```python
from build123d import *

# Parameters (mm, degrees)
F1_DEPTH = 7.25
F2_R     = 0.5


with BuildPart() as f1:
    # F0 (on Top) → F1 (new body, symmetric)
    with BuildSketch(Plane.XY):
        with BuildLine():
            ThreePointArc((-6.9704381548, 3.1520615364), (-5, 0), (-6.9704381548, -3.1520615364))
            ThreePointArc((-6.9704381548, -3.1520615364), (-5.4093668761, -5.4093668761), (-3.1520615364, -6.9704381548))
            ThreePointArc((-3.1520615364, -6.9704381548), (0, -5), (3.1520615364, -6.9704381548))
            ThreePointArc((3.1520615364, -6.9704381548), (5.4093668761, -5.4093668761), (6.9704381548, -3.1520615364))
            ThreePointArc((6.9704381548, -3.1520615364), (5, 0), (6.9704381548, 3.1520615364))
            ThreePointArc((6.9704381548, 3.1520615364), (5.4093668761, 5.4093668761), (3.1520615364, 6.9704381548))
            ThreePointArc((3.1520615364, 6.9704381548), (0, 5), (-3.1520615364, 6.9704381548))
            ThreePointArc((-3.1520615364, 6.9704381548), (-5.4093668761, 5.4093668761), (-6.9704381548, 3.1520615364))
        make_face()
    extrude(amount=F1_DEPTH, both=True)

    # F2
    f2_edges = [f1.edges().sort_by_distance(p)[0] for p in [
        (-3.152062, 6.970438, 0),
        (-6.970438, 3.152062, 0),
        (-6.970438, -3.152062, 0),
        (-3.152062, -6.970438, 0),
        (3.152062, -6.970438, 0),
        (6.970438, -3.152062, 0),
        (6.970438, 3.152062, 0),
        (3.152062, 6.970438, 0),
    ]]
    fillet(f2_edges, radius=F2_R)

    # F3 (on Right) → F4 (revolve, cut)
    with BuildSketch(Plane.YZ):
        Polygon((-7.65, 6.0952994616), (-5.65, 7.25), (-7.65, 7.25), align=None)
        Polygon((-5.65, -7.25), (-7.65, -6.0952994616), (-7.65, -7.25), align=None)
    revolve(axis=Axis((0, 0, 0.0045555644), (0, 0, -1)), mode=Mode.SUBTRACT)


solid = f1.part
```
Part model, mm, in its own coordinate system. Give positions to 0.01 mm unless a question says otherwise; leave off trailing zeros. Write each loop counter-clockwise with the first axis right and the second up, starting at its lowest first coordinate (ties: lowest second). Pieces come first, ordered by that corner, then holes. Notation, with made-up numbers: (74.25, 56) -> (125.25, 56) arc R32 cw to (125.25, 87) -> close; hole circle Ø3 at (6, 21.5). An arc over 180 degrees is marked (long way). Put each result on its own line as item: value. Start each with the question number.
Item 1: Pin check, flat tips, straight feed: pin 1 Ø1 at (x, z) = (-2.5, -5) entering from -Y; pin 2 Ø3 at (y, z) = (-4, -1) entering from +X. Stop position of each tip, or through.
Item 2: Wall check: L1, parallel to X at y = 6, z = -3; L2, parallel to X at y = 6.25, z = -5.5; L3, parallel to Y at x = -5.75, z = 3. Give the ranges that are in metal, low to high. Write a range as [from, to].
Item 3: Cut at B-B (x = -1). List the corners of the cut face in (y, z), then the cut area to 3 significant figures.
Item 4: Cut at A-A (y = 0). List the corners of the cut face in (x, z).
Item 5: Pull direction Y, two halves, no side cores. Call faces 1 (the face through (-4.586, 4.524, -6.793)), 2 (the face through (5, 0, 0)), 3 (the face through (-4.5, -4.57, 6.81)): pulls with the +Y half, pulls with the -Y half, needs draft (parallel to the pull), parting line crosses it, or undercut.
Answer list:
1. pin 1: stops at y = -6.67
1. pin 2: stops at x = 6.81
2. L1: x = [-4.75, -2.45], [2.45, 4.75]
2. L2: x = [-4.41, -2.68], [2.68, 4.41]
2. L3: y = [-5.05, -2.17], [2.17, 5.05]
3. outline: (-5.15, -7.25) -> (5.15, -7.25) -> (5.15, 7.25) -> (-5.15, 7.25) -> close
3. area: 149 mm2
4. outline: (-5, -7.25) -> (5, -7.25) -> (5, 7.25) -> (-5, 7.25) -> close
5. face 1: pulls with the +Y half
5. face 2: undercut
5. face 3: pulls with the -Y half
